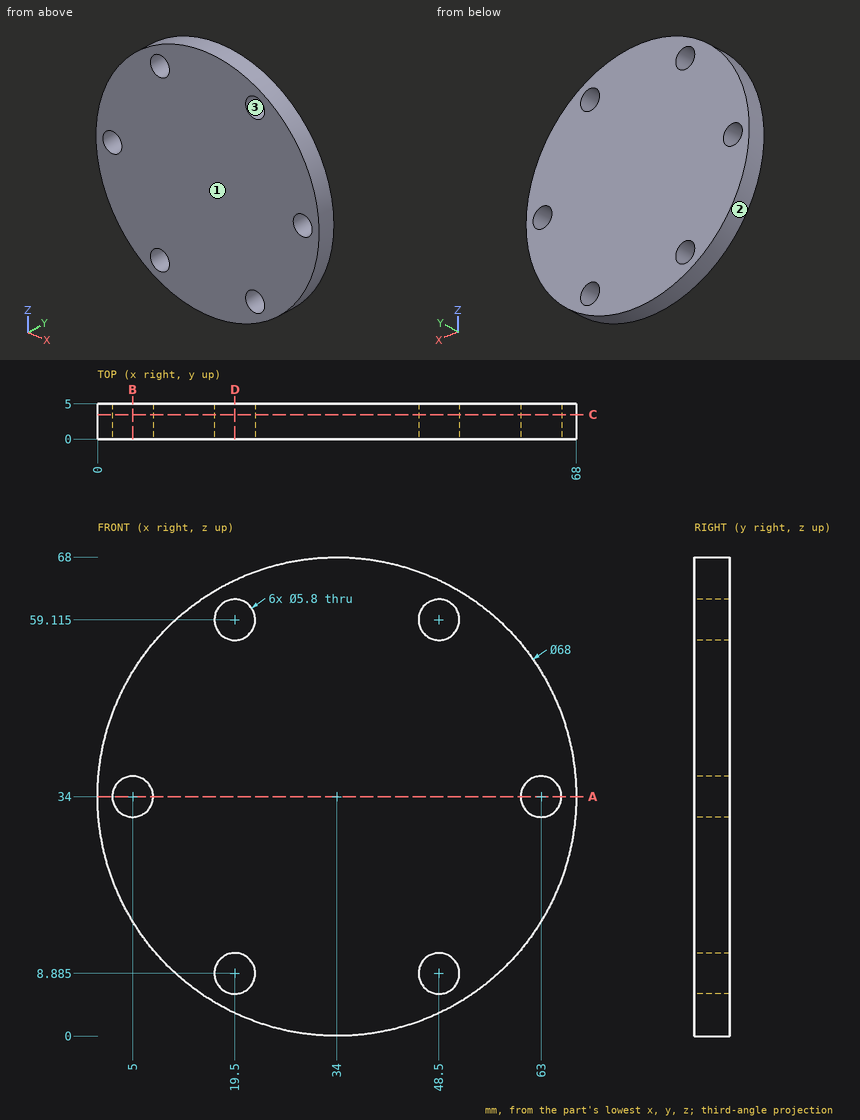
Geometry check sheet. Reference: drawing and pictorial views, mm from the part's lowest x, y, z. Round coordinates to 2 decimals unless told otherwise and drop trailing zeros. Loops run counter-clockwise (first coordinate to the right, second up) from the corner with the lowest first, then second, coordinate; pieces in that order, holes last. Notation, with made-up numbers: (3, 56.5) -> (62, 56.5) arc R17 ccw to (62, 76.5) -> close; hole circle Ø6 at (12.5, 16.5). An arc over 180 degrees is marked (long way). Answer as a JSON object with one key per item and string values. Group by question number.
Item 1: Cross-section at D-D, the plane x = 19.5. Record the cut outline in (y, z) (1 decimal).
Item 2: Thickness scan on line 1 along X through (y, z) = (4.55, 34); line 2 along Z through (x, y) = (18.5, 1.65); line 3 along X through (y, z) = (2.75, 35) (1 decimal). Record the ranges inside material, lowest first.
Item 3: Depth check by flat-ended pin: pin 1 Ø6.5 at (x, z) = (48.5, 59.11) entering from +Y; pin 2 Ø1 at (x, y) = (40, 3.5) entering from +Z. Enter the tip coordinate at first touch or a pass-through.
Item 4: Cross-section at C-C, the plane y = 3.5. Record the cut outline in (x, z) (1 decimal).
Item 5: Cross-section at B-B, the plane x = 5. Record the cut outline in (y, z).
Item 6: Cross-section at A-A, the plane z = 34. Record the cut outline in (x, y), plus the area to 3 significant figures.
Item 7: Release check for a two-part mould opening along Z. For the marked faces 1, 2 and 3 record: pulls with the +Z half, pulls with the -Z half, needs draft (parallel to the pull), parting line crosses it, or undercut.
Determined:
{
 "1": {"outline": "(0, 3.2) -> (5, 3.2) -> (5, 6) -> (0, 6) -> close; (0, 11.8) -> (5, 11.8) -> (5, 56.2) -> (0, 56.2) -> close; (0, 62) -> (5, 62) -> (5, 64.8) -> (0, 64.8) -> close"},
 "2": {"line 1": "x = 0 to 2.1, 7.9 to 60.1, 65.9 to 68", "line 2": "z = 3.74 to 6.16, 11.61 to 56.39, 61.84 to 64.26", "line 3": "x = 0 to 2.3, 7.7 to 60.3, 65.7 to 68"},
 "3": {"pin 1": "stops at y = 5", "pin 2": "stops at z = 67.55"},
 "4": {"outline": "circle Ø68 at (34, 34); hole circle Ø5.8 at (5, 34); hole circle Ø5.8 at (19.5, 8.9); hole circle Ø5.8 at (19.5, 59.1); hole circle Ø5.8 at (48.5, 8.9); hole circle Ø5.8 at (48.5, 59.1); hole circle Ø5.8 at (63, 34)"},
 "5": {"outline": "(0, 16.25) -> (5, 16.25) -> (5, 31.1) -> (0, 31.1) -> close; (0, 36.9) -> (5, 36.9) -> (5, 51.75) -> (0, 51.75) -> close"},
 "6": {"outline": "(0, 0) -> (2.1, 0) -> (2.1, 5) -> (0, 5) -> close; (7.9, 0) -> (60.1, 0) -> (60.1, 5) -> (7.9, 5) -> close; (65.9, 0) -> (68, 0) -> (68, 5) -> (65.9, 5) -> close", "area": "282 mm²"},
 "7": {"face 1": "needs draft", "face 2": "parting line crosses it", "face 3": "undercut"}
}
